Read the model definition and answer for the solid it produces. Units are mm, in the model's axes. Coordinates: 2 decimals unless noted, no trailing zeros. Order: outer loops, then holes, each group sorted by start corner. A loop starts at its lowest first (then second) coordinate and runs counter-clockwise, first axis right, second up. Notation, with made-up numbers: (11, 64.25) - (53, 64.25) arc R27 ccw to (53, 94.25) - close; hole circle Ø2 at (-38, 41.5). An arc over 180 degrees is marked (long way). Write item = value, one per line.
from build123d import *

# Parameters (mm, degrees)
AUFSATZ_LINEAR_AUSTRAGEN1_DEPTH      = 14
AUFSATZ_LINEAR_AUSTRAGEN1_DEPTH_BACK = 14
SKIZZE1_R                            = 10.5
SKIZZE1_R_2                          = 7
FASE1_SIZE                           = 0.2


with BuildPart() as part:
    # Skizze1 → Aufsatz-Linear austragen1 (new, two sides: drawn at the far end of the back side and taken through both)
    with BuildSketch(Plane(origin=(0, 0, 0), x_dir=(1, 0, 0), z_dir=(0, 1, 0)).offset(-AUFSATZ_LINEAR_AUSTRAGEN1_DEPTH_BACK)):
        with Locations(Location((0, 0, 0), (0, 0, 270))):
            Circle(SKIZZE1_R)
        with Locations(Location((0, 0, 0), (0, 0, 270))):
            Circle(SKIZZE1_R_2, mode=Mode.SUBTRACT)
    extrude(amount=AUFSATZ_LINEAR_AUSTRAGEN1_DEPTH + AUFSATZ_LINEAR_AUSTRAGEN1_DEPTH_BACK)

    # Fase1
    fase1_edges = [part.edges().sort_by_distance(p)[0] for p in [
        (0, -14, -10.5),
        (0, -14, -7),
        (0, 14, -10.5),
        (0, 14, -7),
    ]]
    chamfer(fase1_edges, length=FASE1_SIZE)


solid = part.part
1) Flat-ended cylindrical pins translate along their axes: pin 1 Ø1 at (y, z) = (8.5, 6.5) entering from +X; pin 2 Ø4 at (x, y) = (6, -8) entering from +Z; pin 3 Ø2 at (y, z) = (6, -8) entering from -X; pin 4 Ø4 at (y, z) = (3, 0.5) entering from -X. Find the tip coordinate at first contact, or state that the pin passes through.
Returned:
pin_1 = 8.62
pin_2 = 9.71
pin_3 = -7.83
pin_4 = -10.5
2) The part is cut by section C-C (y = 0.5). Determine the outline of the cut face in (x, z), and give its area (3 significant figures).
Returned:
outline = circle Ø21 at (0, 0); hole circle Ø14 at (0, 0)
area = 192 mm^2
3) Straight lines are drawn through the part: line 1 along X through (y, z) = (-3.5, 0); line 2 along Z through (x, y) = (-2.5, -4.25); line 3 along Z through (x, y) = (-4, 6). For each, find the intervals that lie inside material, in ascending order. Write a range as from..to.
Returned:
line_1 = -10.5..-7, 7..10.5
line_2 = -10.2..-6.54, 6.54..10.2
line_3 = -9.71..-5.74, 5.74..9.71
4) The part is cut by section B-B (x = 0). Determine the outline of the cut face in (y, z).
Returned:
outline = (-14, -10.3) - (-13.8, -10.5) - (13.8, -10.5) - (14, -10.3) - (14, -7.2) - (13.8, -7) - (-13.8, -7) - (-14, -7.2) - close; (-14, 7.2) - (-13.8, 7) - (13.8, 7) - (14, 7.2) - (14, 10.3) - (13.8, 10.5) - (-13.8, 10.5) - (-14, 10.3) - close
5) The part is cut by section A-A (z = 0). Determine the outline of the cut face in (x, y), and give its area (3 significant figures).
Returned:
outline = (-10.5, -13.8) - (-10.3, -14) - (-7.2, -14) - (-7, -13.8) - (-7, 13.8) - (-7.2, 14) - (-10.3, 14) - (-10.5, 13.8) - close; (7, -13.8) - (7.2, -14) - (10.3, -14) - (10.5, -13.8) - (10.5, 13.8) - (10.3, 14) - (7.2, 14) - (7, 13.8) - close
area = 196 mm^2
6) Determine the mould class of faces 1 (the face through (3.2, -0.2, 10)), 2 (the face through (7, -14, -2.4)), 3 (the face through (-6.834, -0.193, -1.517)) for opening direction X: pulls with the +X half, pulls with the -X half, needs draft (parallel to the pull), parting line crosses it, or undercut.
Returned:
face_1 = parting line crosses it
face_2 = needs draft
face_3 = undercut
